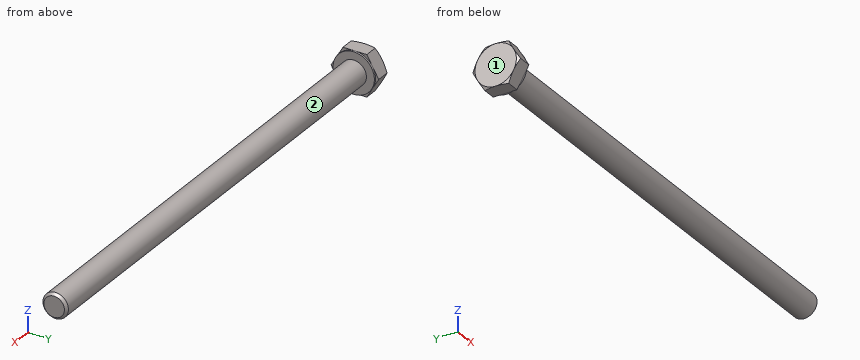
Autodesk Inventor part; units mm, degrees
ref_plane "Work Plane1" through (1.525, 0, 0) normal (0, 0, 1) x (1, 0, 0)
ref_plane "YZ Plane" through (0, 0, 0) normal (1, 0, 0) x (0, 1, 0)
ref_plane "XZ Plane" through (0, 0, 0) normal (0, 1, 0) x (-1, 0, 0)
sketch "Sketch1" plane through (0, 0, 0) normal (0, 0, 1) x (1, 0, 0)
  line L0 (0, 6.5) -> (0, 4)
  line L1 (73.7, 4) -> (150, 4)
  line L2 (150, 4) -> (150, 0)
  line L3 (150, 0) -> (-0.6001, 0)
  line L4 (-30.7201, 0) -> (180.12, 0)
  line L5 (-0.6001, 0) -> (-0.6001, 6.5)
  line L6 (-0.6001, 6.5) -> (0, 6.5)
  line L7 (73.7, 4) -> (72.9331, 4)
  line L8 (72.9331, 4) -> (0, 4)
  line L9 (0, -1.3) -> (0, 7.8)
  dimension "d0" = 150
  dimension "d1" = 76.3
  dimension "d2" = 8
  dimension "d9" = 0.6001
  dimension "d10" = 13
  dimension "d13" = 0.7669
  dimension "d14" = 8
revolve "Body" add sketch "Sketch1" angle 360 about axis through (150, 0, 0) along (-1, 0, 0)
sketch "Sketch2" plane through (-0.6001, 0, 0) normal (-1, 0, 0) x (0, 0, 1)
  line L0 (0, 7.5056) -> (6.5, 3.7528)
  line L1 (6.5, 3.7528) -> (6.5, -3.7528)
  line L2 (6.5, -3.7528) -> (0, -7.5056)
  line L3 (0, -7.5056) -> (-6.5, -3.7528)
  line L4 (-6.5, -3.7528) -> (-6.5, 3.7528)
  line L5 (-6.5, 3.7528) -> (0, 7.5056)
  point P0 (0, 0)
  point P1 (0, 0)
  dimension "d11" = 13
extrude "Head" add sketch "Sketch2" along normal blind 4.7
sketch "Sketch4" plane through (0, 0, 0) normal (0, 0, 1) x (1, 0, 0)
  line L0 (-5.3001, 6.5) -> (-5.3001, 7.5056)
  line L1 (-5.3001, 7.5056) -> (-4.7195, 7.5056)
  line L2 (-4.7195, 7.5056) -> (-5.3001, 6.5)
  line L3 (-6.2401, 0) -> (0.3399, 0)
  line L4 (-0.6001, 7.5056) -> (-5.3001, 7.5056)
  line L5 (-5.3001, 3.7528) -> (-5.3001, 7.5056)
  dimension "d5" = 30
  dimension "d19" = 13
revolve "Chamfer1" cut sketch "Sketch4" angle 360 about axis through (-10, 0, 0) along (1, 0, 0)
thread "Thread"
chamfer "Chamfer2" distance 0.7668 distance2 0.7669 1 edges at (150, -4, 0) measured on face at (150, 0.998, -0.8842)
ref_plane "Work Plane1" through (1.525, 0, 0) normal (0, 0, 1) x (1, 0, 0)
equation "\"d1\" = GEL"
equation "\"d2\" = GD"
equation "\"d10\" = SD2"
equation "\"d14\" = BDM"
equation "\"d11\" = SW"
equation "\"d3\" = KOH - SD"
equation "\"d5\" = ANG1"
equation "\"d19\" = SW0"
equation "\"d15\" = GEL"
equation "\"d6\" = -0.5 * SPD + 0.5 * GD"
equation "\"GD\" = NND"
equation "\"BDM\" = NND"
equation "\"KOH\" = 5.3"
equation "\"GEL\" = 76.3"
equation "\"SW\" = 13"
equation "\"SW0\" = SW"
equation "\"SPD\" = NND - 1.2269 * PTC"
equation "\"SD2\" = SW"
equation "\"SD\" = 0.6"
equation "\"ANG1\" = 30deg"
equation "\"GAL\" = 0.61345 * PTC"
equation "\"GUL\" = 0.61345 * PTC"
equation "\"RR\" = 0.4"
equation "\"WFT\" = SD"
equation "\"GD1\" = THREADDIA - 1.2269 * PTC"
equation "\"THREADDIA\" = 8"
equation "\"SDH\" = SW"
equation "\"TOA\" = 30deg"
equation "\"FAWI\" = 45deg"
equation "\"PTC\" = 1.25"
equation "\"NND\" = 8"
equation "\"E0\" = 1.155 * SW"
properties part number "AS 1110 - M8 x 80" material "Steel, Mild"
Could you check a few things on this model? Use its own coordinates, in mm. Face numbers are marked on the shaded views. A direction names the side the tool comes from. Give positions to 0.01 mm unless a question says otherwise; leave off trailing zeros. Loops run counter-clockwise (first coordinate to the right, second up) from the corner with the lowest first, then second, coordinate; pieces in that order, holes last. Notation, with made-up numbers: (-0.5, 70) - (12.5, 70) arc R14 cw to (12.5, 88) - close; hole circle Ø4 at (-39, 40). An arc over 180 degrees is marked (long way). Answer in a Markdown table with one row per item. Add a question column.
Q1. For pin 1 (1.5 mm diameter, centred on x = 34.5, z = -2.5, fed in from -Y); pin 2 (4 mm diameter, centred on x = 56.5, y = -3, fed in from -Z); pin 3 (6 mm diameter, centred on x = 21, y = 0.5, fed in from +Z), each with a flat end and sliding along its axis, tell me the tip position at first contact or that it passes through.
Q2. Which directions (+Z, -Z, +X, -X, +Y, -Y) give clear straight access to the entire face, cutting with the end or side of a thin tool? Please do the marked faces 1 and 2.
Q3. Please list where these lines run through material, in increasing order: L1, parallel to X at y = 5, z = -2.25; L2, parallel to Z at x = 85, y = 0; L3, parallel to Y at x = 122, z = 1.75. Write a range as from..to.
Q4. If we section it at A-A (x = 11.5): List the corners of the cut face in (y, z) for me.
The answers:
| question | item | result |
|---|---|---|
| 1 | pin 1 | stops at y = -3.6 |
| 1 | pin 2 | stops at z = -3.87 |
| 1 | pin 3 | stops at z = 4 |
| 2 | face 1 | +Z, -Z, -X, +Y, -Y |
| 2 | face 2 | +X |
| 3 | L1 | x = -5.3..0 |
| 3 | L2 | z = -4..4 |
| 3 | L3 | y = -3.6..3.6 |
| 4 | outline | circle Ø8 at (0, 0) |
